Could you check a few things on this model? Use its own coordinates, in mm. Face numbers are marked on the shaded views. Round coordinates to 2 decimals unless told otherwise and drop trailing zeros. Loops run counter-clockwise (first coordinate to the right, second up) from the corner with the lowest first, then second, coordinate; pieces in that order, holes last. Notation, with made-up numbers: (39, 64.25) -> (68, 64.25) arc R25 cw to (68, 89.25) -> close; hole circle Ø11 at (5.25, 39.25). An arc over 180 degrees is marked (long way). One line per item, written item: value.
from build123d import *


with BuildPart() as f1:
    # F0 (on Front) → F1 (revolve)
    with BuildSketch(Plane.XZ):
        with BuildLine():
            Line((1.247333, 16), (0, 16))
            Line((0, 16), (0, 13))
            Line((0, 13), (12, 13))
            Line((12, 13), (12, 11))
            Line((12, 11), (13, 11))
            Line((13, 11), (13, 16))
            Line((13, 16), (12, 16))
            Line((12, 16), (11.749817, 16))
            Line((11.749817, 16), (11.749817, 15.925313))
            ThreePointArc((11.749817, 15.925313), (11.75, 15.9), (11.749817, 15.874687))
            ThreePointArc((11.749817, 15.874687), (9.979433, 14.150121), (8.250072, 15.91582))
            Line((8.250072, 15.91582), (8.250072, 16))
            Line((8.250072, 16), (4.75, 16))
            Line((4.75, 16), (4.75, 15.9))
            ThreePointArc((4.75, 15.9), (3.019522, 14.150109), (1.250436, 15.860959))
            Line((1.250436, 15.860959), (1.247333, 16))
        make_face()
    revolve(axis=Axis((8.760135, 0, 0), (1, 0, 0)))


solid = f1.part
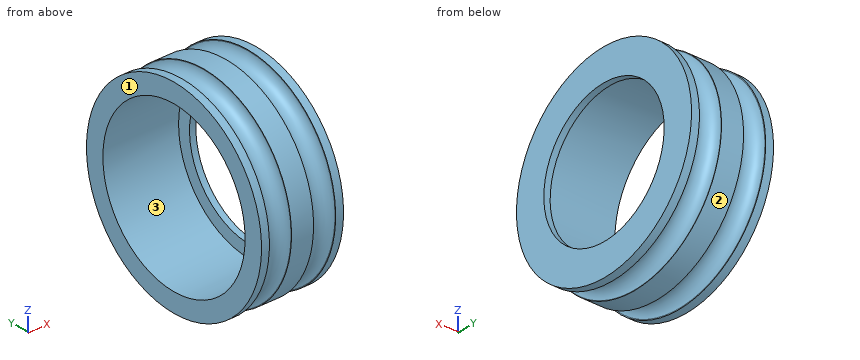
(1) Thinking about a two-plate mould opening in Z: for the marked faces 1, 2 and 3, which applies, released by +Z, released by -Z, zero draft, split by the parting line, or undercut?
Recorded:
face 1: zero draft
face 2: split by the parting line
face 3: undercut
(2) I'm going to push flat-ended pins straight in: pin 1 Ø13 at (y, z) = (2, 2) entering from -X; pin 2 Ø6 at (x, y) = (1.5, 12.5) entering from -Z; pin 3 Ø4 at (x, z) = (3, 12) entering from +Y; pin 4 Ø4 at (x, z) = (3, 11.5) entering from -Y (3 decimals). Where does each tip first touch, or does it pass through?
Recorded:
pin 1: through
pin 2: z = -12.87
pin 3: y = 11.59
pin 4: y = -12.045
(3) If we section it at C-C, the plane x = 7.25: Please give me the cut outline in (y, z), then the cut area to 3 significant figures.
Recorded:
outline: circle Ø32 at (0, 0); hole circle Ø26 at (0, 0)
area: 273 mm²
(4) If I drill on L1, parallel to Z at x = 12.7, y = 0; L2, parallel to X at y = -0.5, z = 11.5, over which ranges is the centre line in solid material (lowest first)?
Recorded:
L1: -16 to -11, 11 to 16
L2: 12 to 13
(5) If we section it at D-D, the plane x = 10.75: Please give me the cut outline in (y, z), then the cut area to 3 significant figures.
Recorded:
outline: circle Ø28.64 at (0, 0); hole circle Ø26 at (0, 0)
area: 113 mm²
